Build history of the part. All positions in model axes, mm. Face numbers are marked on the shaded views. A direction names the side the tool comes from. Round coordinates to 2 decimals unless told otherwise and drop trailing zeros. Order: outer loops, then holes, each group sorted by start corner. A loop starts at its lowest first (then second) coordinate and runs counter-clockwise, first axis right, second up. Notation, with made-up numbers: M 70.5,19 L 97.5,19 A26 ccw 97.5,47 Z; hole C 0.25,74.5 d11. An arc over 180 degrees is marked long. Use CSV: the item, a comma, the result in double quotes.
from build123d import *

# Parameters (mm, degrees)
BOSS_EXTRUDE1_DEPTH            = 100
BOSS_EXTRUDE2_START            = 15
BOSS_EXTRUDE2_DEPTH            = 15
CUT_EXTRUDE1_REACH             = 129.299
CUT_EXTRUDE1_DIRECTION_2_DEPTH = 128.298860953
BOSS_EXTRUDE3_DEPTH            = 10
BOSS_EXTRUDE3_DEPTH_BACK       = 110
SKETCH5_W                      = 20
SKETCH5_H                      = 15
CUT_EXTRUDE2_DEPTH             = 136.295971854
CUT_EXTRUDE2_DEPTH_BACK        = 136.295971854
SKETCH6_W                      = 29
SKETCH6_H                      = 40
FILLET1_R                      = 10


with BuildPart() as part:
    # Sketch1 → Boss-Extrude1 (new body)
    with BuildSketch(Plane.XY):
        with BuildLine():
            Line((10, -35.129619486), (10, -15))
            Line((10, -15), (-30, -15))
            Line((-30, -15), (-30, 0))
            Line((-30, 0), (0, 0))
            Line((0, 0), (0, 66))
            ThreePointArc((0, 66), (42.742771868, 19.167308707), (10, -35.129619486))
        make_face()
    extrude(amount=BOSS_EXTRUDE1_DEPTH)

    # Sketch2 → Boss-Extrude2 (add)
    with BuildSketch(Plane(origin=(0, 0, 0), x_dir=(-1, 0, 0), z_dir=(0, 0, -1)).offset(BOSS_EXTRUDE2_START)):
        with BuildLine():
            Line((30, -15), (30, -10.52909236))
            Line((30, -10.52909236), (-42.207179875, 4.819017522))
            ThreePointArc((-42.207179875, 4.819017522), (-31.260666573, -19.313012165), (-10, -35.129619486))
            Line((-10, -35.129619486), (-10, -15))
            Line((-10, -15), (30, -15))
        make_face()
    extrude(amount=-BOSS_EXTRUDE2_DEPTH)

    # Sketch4 → Cut-Extrude1 (cut, up to next)
    with BuildSketch(Plane(origin=(0, 0, 0), x_dir=(1, 0, 0), z_dir=(0, 1, 0)), mode=Mode.PRIVATE) as cut_extrude1_sk1:
        with BuildLine():
            Line((-20, -10), (-20, -90))
            ThreePointArc((-20, -90), (-15, -95), (-10, -90))
            Line((-10, -90), (-10, -10))
            ThreePointArc((-10, -10), (-15, -5), (-20, -10))
        make_face()
    cut_extrude1_tool1 = extrude(cut_extrude1_sk1.sketch, amount=-CUT_EXTRUDE1_REACH, mode=Mode.PRIVATE) & part.part
    add(cut_extrude1_tool1.solids().sort_by_distance((-15, 0, 50))[0], mode=Mode.SUBTRACT)

    # Sketch4 → Cut-Extrude1 direction 2 (cut)
    with BuildSketch(Plane(origin=(0, 0, 0), x_dir=(1, 0, 0), z_dir=(0, 1, 0))):
        with BuildLine():
            Line((-20, -10), (-20, -90))
            ThreePointArc((-20, -90), (-15, -95), (-10, -90))
            Line((-10, -90), (-10, -10))
            ThreePointArc((-10, -10), (-15, -5), (-20, -10))
        make_face()
    extrude(amount=CUT_EXTRUDE1_DIRECTION_2_DEPTH, mode=Mode.SUBTRACT)

    # Sketch5 → Boss-Extrude3 (add, two sides: drawn at the far end of the back side and taken through both)
    with BuildSketch(Plane.XY.offset(100).offset(-BOSS_EXTRUDE3_DEPTH_BACK)):
        with Locations((5, 43.5)):
            Rectangle(SKETCH5_W, SKETCH5_H)
    extrude(amount=BOSS_EXTRUDE3_DEPTH + BOSS_EXTRUDE3_DEPTH_BACK)

    # Sketch6 → Cut-Extrude2 (cut, two sides: drawn at the far end of the back side and taken through both)
    with BuildSketch(Plane.ZY.offset(-CUT_EXTRUDE2_DEPTH_BACK)):
        with Locations((44.5, 46)):
            Rectangle(SKETCH6_W, SKETCH6_H)
    extrude(amount=CUT_EXTRUDE2_DEPTH + CUT_EXTRUDE2_DEPTH_BACK, mode=Mode.SUBTRACT)

    # Fillet1
    fillet1_edges = [part.edges().sort_by_distance(p)[0] for p in [
        (0, 0, 50),
    ]]
    fillet(fillet1_edges, radius=FILLET1_R - 0.0001)  # a hair under: the kernel refuses the full size


solid = part.part
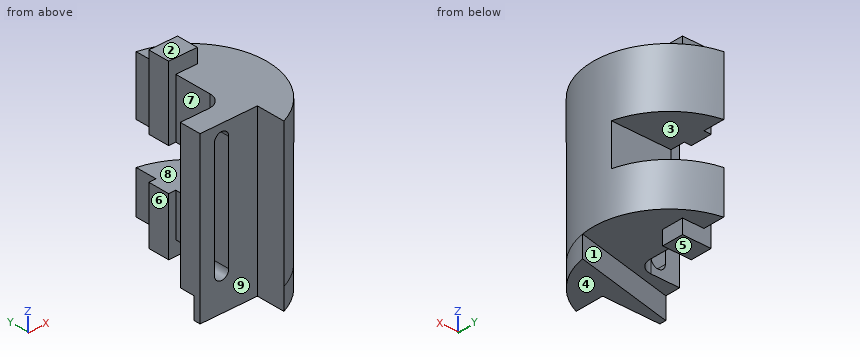
(1) Cut at C-C, the plane y = 49. Give the cut face in (x, z), and give its area (3 significant figures).
Answer block:
outline,"M -5,-10 L 15,-10 L 15,0 L 29.76,0 L 29.76,30 L -5,30 Z; M -5,59 L 29.76,59 L 29.76,100 L 15,100 L 15,110 L -5,110 Z"
area,"2,870 mm²"
(2) Cut at D-D, the plane z = 96.5. Give the cut face in (x, y).
Answer block:
outline,"M -30,-15 L 10,-15 L 10,-35.13 A53 ccw 0,66 L 0,51 L -5,51 L -5,36 L 0,36 L 0,10 A10 cw -10,0 L -30,0 Z"
(3) Wall check: line 1 (Z direction, x = 16, y = 31); line 2 (Y direction, x = -22.5, z = 17); line 3 (Z direction, x = 28.5, y = -16). Give the ranges that are in metal, low to high. Write a range as from..to.
Answer block:
line 1,"z = 0..30, 59..100"
line 2,"y = -15..0"
line 3,"z = -15..100"
(4) Two-plate mould, pull along Z, no slides. Class the marked faces 1, 2, 3 and 4: released by +Z, released by -Z, zero draft, split by the parting line, or undercut.
Answer block:
face 1,"zero draft"
face 2,"released by +Z"
face 3,"undercut"
face 4,"released by -Z"
(5) Cut at B-B, the plane x = -15. Give the cut face in (y, z), and give its area (3 significant figures).
Answer block:
outline,"M -15,-15 L -7.34,-15 L -7.34,0 L 0,0 L 0,5 L -15,5 Z; M -15,95 L 0,95 L 0,100 L -15,100 Z"
area,"265 mm²"
(6) Drop flat-ended pins along their axis: pin 1 (4 mm diameter, centred on x = 13, y = 19, fed in from -Z); pin 2 (4 mm diameter, centred on y = 34.5, z = 75, fed in from -X); pin 3 (4 mm diameter, centred on x = 34, z = 84.5, fed in from -Y). Give the stop position or say it passes through.
Answer block:
pin 1,"stops at z = 0"
pin 2,"stops at x = -5"
pin 3,"stops at y = -18.37"
(7) Tool access for the marked faces 5, 6, 7, 8 and 9: list every direction of +Z, -Z, +X, -X, +Y, -Y with a clear straight run to the whole face (end or side of a thin tool).
Answer block:
face 5,"-Z, +X, -X, +Y"
face 6,"+Z, -Z, -X, +Y"
face 7,"+Z, -Z, -X"
face 8,"+X, -X, +Y"
face 9,"+Z, -Z, -X, -Y"
